The listing builds one solid part. Answer for the finished solid, in the listing's coordinates (mm). Face numbers are marked on the shaded views. A direction names the side the tool comes from. Round coordinates to 2 decimals unless told otherwise and drop trailing zeros. Order: outer loops, then holes, each group sorted by start corner. A loop starts at its lowest first (then second) coordinate and runs counter-clockwise, first axis right, second up. Notation, with made-up numbers: M 18.5,68 L 64.5,68 A23 cw 64.5,77 Z; hole C 83,70 d1. An arc over 180 degrees is marked long. Write item = value, one per line. Start each with the question number.
(1) A cutting plane is placed at D-D, the plane x = 15.5. Determine the outline of the cut face in (y, z), and give its area (3 significant figures).
(2) A cutting plane is placed at B-B, the plane z = 3.5. Determine the outline of the cut face in (x, y), and give its area (3 significant figures).
(3) Each of these flat-tipped pins is pushed along its axis until it touches: pin 1 (1 mm diameter, centred on y = -10.5, z = 3, fed in from -X); pin 2 (17.5 mm diameter, centred on x = 22, y = -12.7, fed in from +Z); pin 3 (2 mm diameter, centred on y = -14, z = 2, fed in from -X). Where does it stop, or does it pass through?
(4) A cutting plane is placed at A-A, the plane y = 30. Determine the outline of the cut face in (x, z).
(5) Which of the six approach directions +Z, -Z, +X, -X, +Y, -Y give full straight-line access (tool end or side, diameter ignored) to the marked faces 1 and 2?
(6) Straight lines are drawn through the part: probe 1 along X at (y, z) = (-12.7, 3.5); probe 2 along Y at (x, z) = (0.5, 7); probe 3 along Y at (x, z) = (7.5, 6.75). For each, find the intervals that lie inside material, in ascending order. Write a range as from..to.
(7) A cutting plane is placed at C-C, the plane y = -5. Determine the outline of the cut face in (x, z).
(8) For a pull along Y with two mould halves and no side action, classify the marked faces 3, 4 and 5 as released by +Y, released by -Y, zero draft, split by the parting line, or undercut.
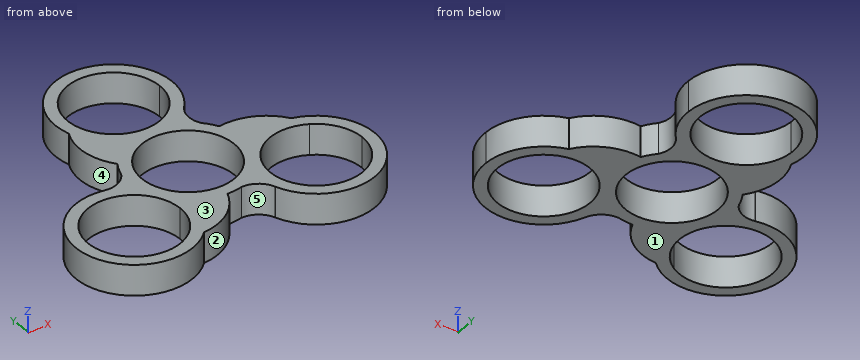
from build123d import *

# Parameters (mm, degrees)
F0_R     = 11.049
F1_DEPTH = 7.2898


# Not quite as in the source:
# - a feature names something its author has since deleted; it is built from what else it names


with BuildPart() as f1:
    # F0 (on Top) → F1 (new body)
    with BuildSketch(Plane.XY):
        with BuildLine():
            ThreePointArc((13.9084581944, -1.3098437524), (13.9546060671, -0.655644349), (13.97, 0))
            ThreePointArc((13.97, 0), (13.5399902372, 3.4394133768), (12.2764331601, 6.6670899848))
            ThreePointArc((12.2764331601, 6.6670899848), (11.2762217496, 8.2466795168), (10.0740419848, 9.6785628111))
            ThreePointArc((10.0740419848, 9.6785628111), (8.0892761862, 11.3896668425), (5.8198711326, 12.7))
            ThreePointArc((5.8198711326, 12.7), (0, 11.43), (-5.8198711326, 12.7))
            ThreePointArc((-5.8198711326, 12.7), (-9.2682549118, 10.4527676187), (-11.9120858762, 7.2981579921))
            ThreePointArc((-11.9120858762, 7.2981579921), (-12.7799448333, 5.6421547355), (-13.4189022589, 3.8850948721))
            ThreePointArc((-13.4189022589, 3.8850948721), (-13.9083789193, 1.3106852543), (-13.9084581944, -1.3098437524))
            ThreePointArc((-13.9084581944, -1.3098437524), (-9.8986703653, -5.715), (-8.0885870618, -11.3901562476))
            ThreePointArc((-8.0885870618, -11.3901562476), (-4.4182348417, -13.2529280117), (-0.3643472839, -13.9652479769))
            ThreePointArc((-0.3643472839, -13.9652479769), (1.5037230836, -13.8888342523), (3.3448602741, -13.5636576832))
            ThreePointArc((3.3448602741, -13.5636576832), (5.8191027331, -12.7003520968), (8.0885870618, -11.3901562476))
            ThreePointArc((8.0885870618, -11.3901562476), (9.8986703653, -5.715), (13.9084581944, -1.3098437524))
        make_face()
        Circle(F0_R, mode=Mode.SUBTRACT)
        with BuildLine():
            ThreePointArc((12.2764331601, 6.6670899848), (13.5399902372, 3.4394133768), (13.97, 0))
            ThreePointArc((13.97, 0), (13.9546060671, -0.655644349), (13.9084581944, -1.3098437524))
            ThreePointArc((13.9084581944, -1.3098437524), (19.4758239296, 1.0406092668), (25.5149823418, 0.8198009845))
            ThreePointArc((25.5149823418, 0.8198009845), (19.7483617265, 5.673895919), (12.2764331601, 6.6670899848))
        make_face()
        with BuildLine():
            ThreePointArc((25.5149823418, 0.8198009845), (19.4758239296, 1.0406092668), (13.9084581944, -1.3098437524))
            ThreePointArc((13.9084581944, -1.3098437524), (12.0983748909, -6.985), (8.0885870618, -11.3901562476))
            ThreePointArc((8.0885870618, -11.3901562476), (8.1283324688, -14.3791979101), (8.8030929872, -17.2913531259))
            ThreePointArc((8.8030929872, -17.2913531259), (8.8153498636, -17.3259186272), (8.8273812481, -17.3605632616))
            ThreePointArc((8.8273812481, -17.3605632616), (24.3614367008, -26.4684622633), (35.9670452561, -12.7))
            ThreePointArc((35.9670452561, -12.7), (33.0493409698, -4.1555480306), (25.5149823418, 0.8198009845))
        make_face()
        with BuildLine():
            ThreePointArc((33.0460452561, -12.7), (12.502346623, -18.3507609104), (27.2661377773, -2.9883026713))
            ThreePointArc((27.2661377773, -2.9883026713), (31.4917438892, -7.0492390896), (33.0460452561, -12.7))
        make_face(mode=Mode.SUBTRACT)
        with BuildLine():
            ThreePointArc((8.0885870618, -11.3901562476), (12.0983748909, -6.985), (13.9084581944, -1.3098437524))
            ThreePointArc((13.9084581944, -1.3098437524), (9.8986703653, -5.715), (8.0885870618, -11.3901562476))
        make_face()
        with BuildLine():
            ThreePointArc((5.8198711326, 12.7), (8.0892761862, 11.3896668425), (10.0740419848, 9.6785628111))
            ThreePointArc((10.0740419848, 9.6785628111), (9.2542217215, 13.054963054), (10.5732045792, 16.2693787218))
            ThreePointArc((10.5732045792, 16.2693787218), (8.3885844419, 14.2289413634), (5.8198711326, 12.7))
        make_face()
        with BuildLine():
            ThreePointArc((8.8030929872, -17.2913531259), (8.1283324688, -14.3791979101), (8.0885870618, -11.3901562476))
            ThreePointArc((8.0885870618, -11.3901562476), (5.8191027331, -12.7003520968), (3.3448602741, -13.5636576832))
            ThreePointArc((3.3448602741, -13.5636576832), (6.6788187895, -14.54187263), (8.8030929872, -17.2913531259))
        make_face()
        with BuildLine():
            ThreePointArc((-5.8198711326, 12.7), (0, 11.43), (5.8198711326, 12.7))
            ThreePointArc((5.8198711326, 12.7), (0, 13.97), (-5.8198711326, 12.7))
        make_face()
        with BuildLine():
            ThreePointArc((-5.8198711326, 12.7), (0, 13.97), (5.8198711326, 12.7))
            ThreePointArc((5.8198711326, 12.7), (8.3885844419, 14.2289413634), (10.5732045792, 16.2693787218))
            ThreePointArc((10.5732045792, 16.2693787218), (10.5970107433, 16.2972762387), (10.6209981845, 16.3250180405))
            ThreePointArc((10.6209981845, 16.3250180405), (13.1060338134, 20.563391924), (13.97, 25.4))
            ThreePointArc((13.97, 25.4), (-1.87356461, 39.2437948429), (-13.4674596495, 21.6867223928))
            ThreePointArc((-13.4674596495, 21.6867223928), (-10.6391060252, 16.3462536492), (-5.8198711326, 12.7))
        make_face()
        with BuildLine():
            ThreePointArc((11.049, 25.4), (0.1463531826, 14.3519693273), (-11.0451228611, 25.1073193139))
            ThreePointArc((-11.0451228611, 25.1073193139), (-0.1463531826, 36.4480306727), (11.049, 25.4))
        make_face(mode=Mode.SUBTRACT)
        with BuildLine():
            ThreePointArc((8.8273812481, -17.3605632616), (8.8153498636, -17.3259186272), (8.8030929872, -17.2913531259))
            ThreePointArc((8.8030929872, -17.2913531259), (8.8151916949, -17.3259741342), (8.8273812481, -17.3605632616))
        make_face()
        with BuildLine():
            ThreePointArc((-11.9120858762, 7.2981579921), (-9.2682549118, 10.4527676187), (-5.8198711326, 12.7))
            ThreePointArc((-5.8198711326, 12.7), (-10.6391060252, 16.3462536492), (-13.4674596495, 21.6867223928))
            ThreePointArc((-13.4674596495, 21.6867223928), (-14.7879188675, 14.2656349788), (-11.9120858762, 7.2981579921))
        make_face()
        with BuildLine():
            ThreePointArc((-12.0475226922, -22.5065233774), (-4.960442859, -19.9395308977), (-0.3643472839, -13.9652479769))
            ThreePointArc((-0.3643472839, -13.9652479769), (-4.4182348417, -13.2529280117), (-8.0885870618, -11.3901562476))
            ThreePointArc((-8.0885870618, -11.3901562476), (-8.042439189, -12.044355651), (-8.0270452561, -12.7))
            ThreePointArc((-8.0270452561, -12.7), (-9.0711849324, -17.9993428735), (-12.0475226922, -22.5065233774))
        make_face()
        with BuildLine():
            ThreePointArc((-8.0270452561, -12.7), (-8.042439189, -12.044355651), (-8.0885870618, -11.3901562476))
            ThreePointArc((-8.0885870618, -11.3901562476), (-12.0983748909, -6.985), (-13.9084581944, -1.3098437524))
            ThreePointArc((-13.9084581944, -1.3098437524), (-16.5169169106, 0.1502565467), (-19.3762975665, 1.0219744041))
            ThreePointArc((-19.3762975665, 1.0219744041), (-19.4123606069, 1.0286423885), (-19.4483794326, 1.0355452211))
            ThreePointArc((-19.4483794326, 1.0355452211), (-35.3240264115, -16.8895671954), (-12.0475226922, -22.5065233774))
            ThreePointArc((-12.0475226922, -22.5065233774), (-9.0711849324, -17.9993428735), (-8.0270452561, -12.7))
        make_face()
        with BuildLine():
            ThreePointArc((-10.9480452561, -12.7), (-12.3559934404, -18.0972697623), (-16.2210149162, -22.1190166425))
            ThreePointArc((-16.2210149162, -22.1190166425), (-31.6380970718, -7.3027302377), (-10.9480452561, -12.7))
        make_face(mode=Mode.SUBTRACT)
        with BuildLine():
            ThreePointArc((-13.9084581944, -1.3098437524), (-12.0983748909, -6.985), (-8.0885870618, -11.3901562476))
            ThreePointArc((-8.0885870618, -11.3901562476), (-9.8986703653, -5.715), (-13.9084581944, -1.3098437524))
        make_face()
        with BuildLine():
            ThreePointArc((-13.9084581944, -1.3098437524), (-13.9083789193, 1.3106852543), (-13.4189022589, 3.8850948721))
            ThreePointArc((-13.4189022589, 3.8850948721), (-15.933040511, 1.486909576), (-19.3762975665, 1.0219744041))
            ThreePointArc((-19.3762975665, 1.0219744041), (-16.5169169106, 0.1502565467), (-13.9084581944, -1.3098437524))
        make_face()
        with BuildLine():
            ThreePointArc((-19.3762975665, 1.0219744041), (-19.412329593, 1.0288071201), (-19.4483794326, 1.0355452211))
            ThreePointArc((-19.4483794326, 1.0355452211), (-19.4123606069, 1.0286423885), (-19.3762975665, 1.0219744041))
        make_face()
    extrude(amount=F1_DEPTH)


solid = f1.part
Reported:
q1.outline = M -25.07,0 L -21.64,0 L -21.64,7.29 L -25.07,7.29 Z; M -3.76,0 L 6.77,0 L 6.77,7.29 L -3.76,7.29 Z
q1.area = 102 mm²
q2.outline = M -19.38,1.02 A13.97 ccw long -12.05,-22.51 A13.46 ccw -0.36,-13.97 A13.97 ccw 3.34,-13.56 A5.63 cw 8.8,-17.29 A13.97 ccw 8.83,-17.36 A13.97 ccw long 25.51,0.82 A13.46 ccw 12.28,6.67 A13.97 ccw 10.07,9.68 A5.63 cw 10.57,16.27 A5.63 cw 10.62,16.33 A13.97 ccw long -13.47,21.69 A13.46 ccw -11.91,7.3 A13.97 ccw -13.42,3.89 A5.63 cw Z; hole C -22,-12.7 d22.1; hole C 0,0 d22.1; hole C 0,25.4 d22.1; hole C 22,-12.7 d22.1
q2.area = 1,050 mm²
q3.pin_1 = -35.86
q3.pin_2 = through
q3.pin_3 = -35.96
q4.outline = M -13.19,0 L -10.05,0 L -10.05,7.29 L -13.19,7.29 Z; M 10.05,0 L 13.19,0 L 13.19,7.29 L 10.05,7.29 Z
q5.face_1 = -Z, +X, -X, +Y, -Y
q5.face_2 = +Z, -Z, -Y
q6.probe_1 = -35.97..-33.05, -10.95..10.95, 33.05..35.97
q6.probe_2 = -13.96..-11.04, 11.04..14.36, 36.44..39.36
q6.probe_3 = -15.23..-8.11, 8.11..17.29, 33.51..37.19
q7.outline = M -33.65,0 L -29.92,0 L -29.92,7.29 L -33.65,7.29 Z; M -14.07,0 L -9.85,0 L -9.85,7.29 L -14.07,7.29 Z; M 9.85,0 L 14.07,0 L 14.07,7.29 L 9.85,7.29 Z; M 29.92,0 L 33.65,0 L 33.65,7.29 L 29.92,7.29 Z
q8.face_3 = zero draft
q8.face_4 = undercut
q8.face_5 = released by -Y
